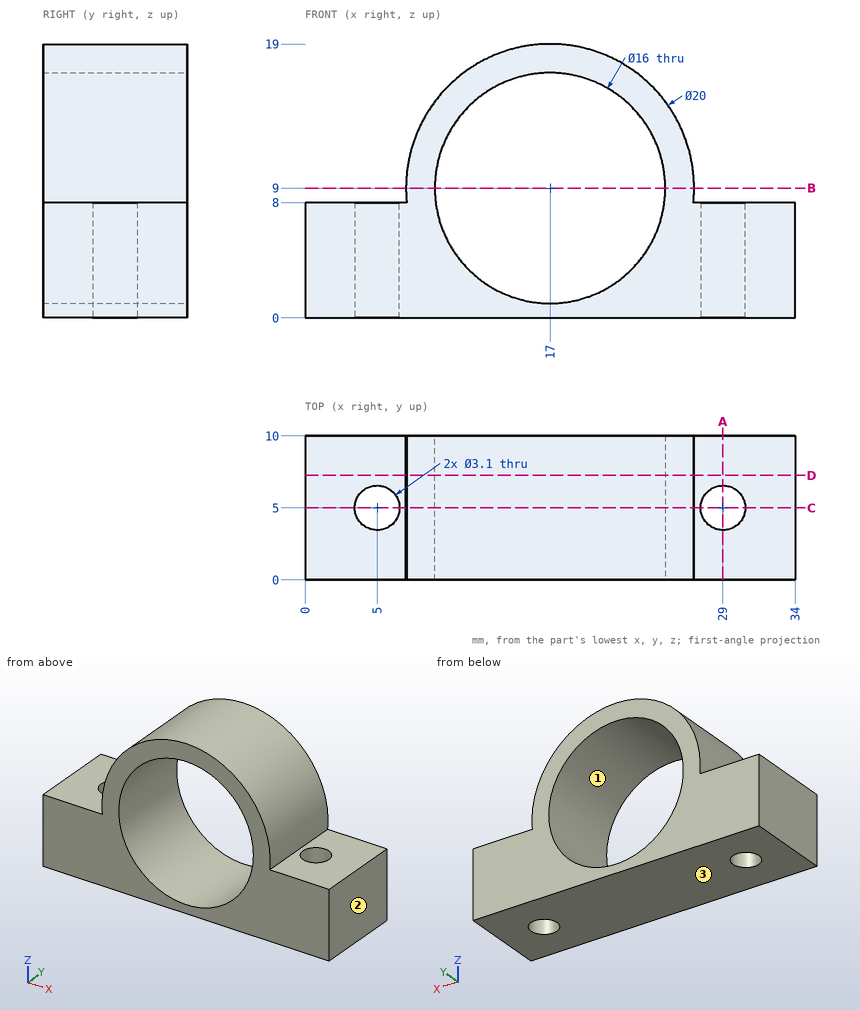
The drawing under review shows one solid part. Ordinate dimensions are in mm from its lowest x, y, z. Give positions to 0.01 mm unless a question says otherwise; leave off trailing zeros. Write each loop counter-clockwise with the first axis right and the second up, starting at its lowest first coordinate (ties: lowest second). Pieces come first, ordered by that corner, then holes. Notation, with made-up numbers: (78.5, -31.75) -> (107.5, -31.75) arc R14 ccw to (107.5, -8.75) -> close; hole circle Ø4 at (39, 9). An arc over 180 degrees is marked (long way). Put each result on its own line as item: value.
(1) To check wall thickness, follow probe 1 along Z at (x, y) = (17, 4.5); probe 2 along X at (y, z) = (6, 4.75); probe 3 along Y at (x, z) = (29, 2.75). State the ranges of each line that lie inside material, in increasing order. Write a range as from..to.
Results are:
probe 1: 0..1, 17..19
probe 2: 0..3.82, 6.18..10.22, 23.78..27.82, 30.18..34
probe 3: 0..3.45, 6.55..10
(2) The part is to be moulded in two halves that separate along Z. For the marked faces 1, 2 and 3, say which applies: pulls with the +Z half, pulls with the -Z half, needs draft (parallel to the pull), parting line crosses it, or undercut.
Results are:
face 1: undercut
face 2: needs draft
face 3: pulls with the -Z half
(3) We need section C-C, the plane y = 5. Give the boundary of the cut face in (x, z), and give its area (3 significant figures).
Results are:
outline: (0, 0) -> (3.45, 0) -> (3.45, 8) -> (0, 8) -> close; (6.55, 0) -> (27.45, 0) -> (27.45, 8) -> (26.95, 8) arc R10 ccw (long way) to (7.05, 8) -> (6.55, 8) -> close; (30.55, 0) -> (34, 0) -> (34, 8) -> (30.55, 8) -> close; hole circle Ø16 at (17, 9)
area: 198 mm²
(4) For pin 1 Ø3 at (x, y) = (19, 8.5) entering from +Z; pin 2 Ø9.5 at (x, z) = (17, 9) entering from -Y; pin 3 Ø3.5 at (x, y) = (30.5, 3.5) entering from +Z; pin 4 Ø2 at (y, z) = (6, 15.5) entering from -X, all flat-tipped, find the tip position at first contact; note any pin that passes through.
Results are:
pin 1: z = 18.99
pin 2: through
pin 3: z = 8
pin 4: x = 8.65
(5) We need section D-D, the plane y = 7.25. Give the boundary of the cut face in (x, z), and give its area (3 significant figures).
Results are:
outline: (0, 0) -> (34, 0) -> (34, 8) -> (26.95, 8) arc R10 ccw (long way) to (7.05, 8) -> (0, 8) -> close; hole circle Ø16 at (17, 9)
area: 248 mm²
(6) We need section B-B, the plane z = 9. Give the boundary of the cut face in (x, y).
Results are:
outline: (7, 0) -> (9, 0) -> (9, 10) -> (7, 10) -> close; (25, 0) -> (27, 0) -> (27, 10) -> (25, 10) -> close
(7) We need section A-A, the plane x = 29. Give the boundary of the cut face in (y, z).
Results are:
outline: (0, 0) -> (3.45, 0) -> (3.45, 8) -> (0, 8) -> close; (6.55, 0) -> (10, 0) -> (10, 8) -> (6.55, 8) -> close
